Print and shaded views of the part. All mm, measured from the part's lowest x, y and z. A direction names the side the tool comes from. Round coordinates to 2 decimals unless told otherwise and drop trailing zeros. Order: outer loops, then holes, each group sorted by start corner. A loop starts at its lowest first (then second) coordinate and runs counter-clockwise, first axis right, second up. Notation, with made-up numbers: (60.5, 71.5) - (115.5, 71.5) arc R15 ccw to (115.5, 83.5) - close; hole circle Ø4 at (70, 35). An arc over 180 degrees is marked (long way). Return JSON: item names as keys, results as strings. Group by question number.
Item 1: Probe probe 1 along X at (y, z) = (25.5, 1.75); probe 2 along Z at (x, y) = (24, 39). List the from-to ranges inside material, lowest first.
Item 2: Tool access for the marked faces 4 and 5: list every direction of +Z, -Z, +X, -X, +Y, -Y with a clear straight run to the whole face (end or side of a thin tool).
Item 3: Drop a flat-ended pin along its axis: pin 1 (6 mm diameter, centred on x = 40, y = 17.5, fed in from +Z). Give the stop position or say it passes through.
Item 4: Two-plate mould, pull along Y, no slides. Class the marked faces 1, 2 and 3: released by +Y, released by -Y, zero draft, split by the parting line, or undercut.
Item 5: Saw through at A-A on z = 2.75. List the corners of the cut face in (x, y).
Item 6: Saw through at B-B on y = 37. List the corners of the cut face in (x, z).
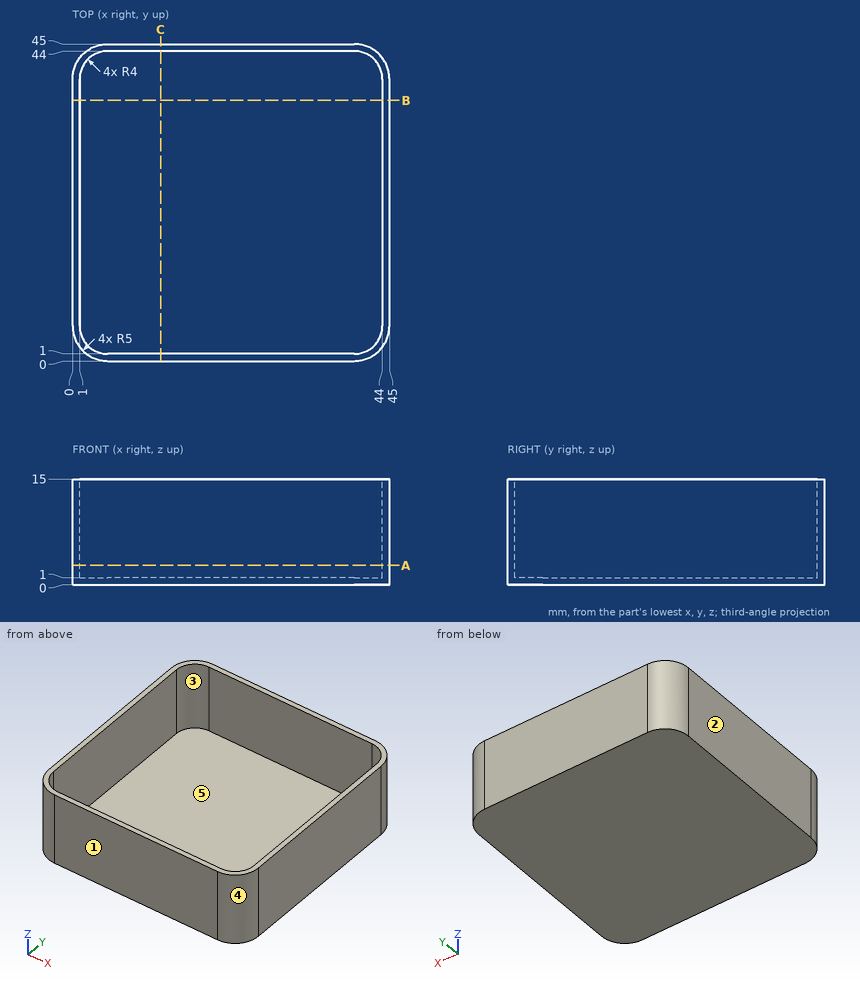
Filled in:
{
 "1": {"probe 1": "x = 0 to 1, 44 to 45", "probe 2": "z = 0 to 1"},
 "2": {"face 4": "+Z, -Z, +X, -Y", "face 5": "+Z"},
 "3": {"pin 1": "stops at z = 1"},
 "4": {"face 1": "released by -Y", "face 2": "zero draft", "face 3": "undercut"},
 "5": {"outline": "(0, 5) arc R5 ccw to (5, 0) - (40, 0) arc R5 ccw to (45, 5) - (45, 40) arc R5 ccw to (40, 45) - (5, 45) arc R5 ccw to (0, 40) - close; hole (1, 5) arc R4 ccw to (5, 1) - (40, 1) arc R4 ccw to (44, 5) - (44, 40) arc R4 ccw to (40, 44) - (5, 44) arc R4 ccw to (1, 40) - close"},
 "6": {"outline": "(0, 0) - (45, 0) - (45, 15) - (44, 15) - (44, 1) - (1, 1) - (1, 15) - (0, 15) - close"}
}
